```python
from build123d import *

# Parameters (mm, degrees)
ESQUISSE2_R                  = 1.5
ENL_V_MAT_EXTRU_1_DEPTH      = 15.5
ENL_V_MAT_EXTRU_1_DEPTH_BACK = 15.5
ESQUISSE3_R                  = 1.5
ENL_V_MAT_EXTRU_2_DEPTH      = 15.5000001
ENL_V_MAT_EXTRU_2_DEPTH_BACK = 15.5000001
CONG_1_R                     = 2
CONG_2_R                     = 1
CHANFREIN1_SIZE              = 1


with BuildPart() as part:
    # Esquisse1 → Révolution1 (revolve)
    with BuildSketch(Plane(origin=(0, 0, 0), x_dir=(0, 0, -1), z_dir=(1, 0, 0))):
        Polygon((-45, 11), (-45, 7), (-50, 7), (-50, 14.5), (50, 14.5), (50, 11), align=None)
    revolve(axis=Axis((0, 0, 50), (0, 0, -1)))

    # Esquisse2 → Enlèv. mat.-Extru.1 (cut, two sides)
    with BuildSketch(Plane(origin=(0, 0, 0), x_dir=(0, 0, -1), z_dir=(1, 0, 0))) as enl_v_mat_extru_1_sk:
        with Locations((39.5, 0)):
            Circle(ESQUISSE2_R)
    extrude(amount=ENL_V_MAT_EXTRU_1_DEPTH, mode=Mode.SUBTRACT)
    extrude(enl_v_mat_extru_1_sk.sketch, amount=-ENL_V_MAT_EXTRU_1_DEPTH_BACK, mode=Mode.SUBTRACT)

    # Esquisse3 → Enlèv. mat.-Extru.2 (cut, two sides)
    with BuildSketch(Plane(origin=(0, 0, 0), x_dir=(1, 0, 0), z_dir=(0, 1, 0))) as enl_v_mat_extru_2_sk:
        with Locations((0, 45.5)):
            Circle(ESQUISSE3_R)
    extrude(amount=ENL_V_MAT_EXTRU_2_DEPTH, mode=Mode.SUBTRACT)
    extrude(enl_v_mat_extru_2_sk.sketch, amount=-ENL_V_MAT_EXTRU_2_DEPTH_BACK, mode=Mode.SUBTRACT)

    # Congé1
    cong_1_edges = [part.edges().sort_by_distance(p)[0] for p in [
        (0, -11, 45),
    ]]
    fillet(cong_1_edges, radius=CONG_1_R)

    # Congé2
    cong_2_edges = [part.edges().sort_by_distance(p)[0] for p in [
        (0, -7, 45),
    ]]
    fillet(cong_2_edges, radius=CONG_2_R)

    # Chanfrein1
    chanfrein1_edges = [part.edges().sort_by_distance(p)[0] for p in [
        (0, -14.5, 50),
        (0, -14.5, -50),
    ]]
    chamfer(chanfrein1_edges, length=CHANFREIN1_SIZE)


solid = part.part
```
The listing builds one solid part. Answer for the finished solid, in the listing's coordinates (mm). A direction names the side the tool comes from. Round coordinates to 2 decimals unless told otherwise and drop trailing zeros. Write each loop counter-clockwise with the first axis right and the second up, starting at its lowest first coordinate (ties: lowest second). Pieces come first, ordered by that corner, then holes. Notation, with made-up numbers: (40.25, -4) -> (91.25, -4) arc R16 ccw to (91.25, 18) -> close; hole circle Ø9 at (-19.75, -13.5). An arc over 180 degrees is marked (long way). Answer as a JSON object with one key per item and string values. Group by question number.
Q1. Which of the six approach directions +Z, -Z, +X, -X, +Y, -Y give full straight-line access (tool end or side, diameter ignored) to faces 5 (the face through (12.7, -0.9, -38.3)), 6 (the face through (-4.213, 10.161, -2.849))?
Q2. Determine the mould class of faces 1 (the face through (-12.7, -0.9, -38.3)), 2 (the face through (-10, -5, -50)), 3 (the face through (0, 13, -44)), 4 (the face through (-6, -6, 50)) for opening direction Z: pulls with the +Z half, pulls with the -Z half, needs draft (parallel to the pull), parting line crosses it, or undercut.
Q3. Each of these flat-tipped pins is pushed along its axis until it touches: pin 1 Ø1.5 at (y, z) = (-8.5, 3) entering from +X; pin 2 Ø1 at (y, z) = (4.5, 26) entering from -X; pin 3 Ø1.5 at (x, z) = (-5, -0.5) entering from +Y. Where does it stop, or does it pass through?
Q4. Section C-C (z = -39.5) is taken. Write down the section's boundary in (x, y), plus the area to 3 significant figures.
Q5. Section A-A (x = 0) is taken. Write down the section's boundary in (y, z), plus the area to 3 significant figures.
Q6. Straight lines are drawn through the part: line 1 along Z through (x, y) = (-7.25, -5); line 2 along Y through (x, z) = (-0.5, -25.5); line 3 along X through (y, z) = (7, 29). For each, find the intervals that lie inside material, in ascending order.
Q7. Section D-D (z = 0.5) is taken. Write down the section's boundary in (x, y).
Q8. Section B-B (y = 0) is taken. Write down the section's boundary in (x, z).
Check values:
{
 "1": {"face 5": "+X, -X", "face 6": "-Z"},
 "2": {"face 1": "undercut", "face 2": "pulls with the -Z half", "face 3": "undercut", "face 4": "pulls with the +Z half"},
 "3": {"pin 1": "x = 12.26", "pin 2": "x = -13.94", "pin 3": "y = 13.86"},
 "4": {"outline": "(-14.42, -1.5) arc R14.5 ccw to (14.42, -1.5) -> (10.9, -1.5) arc R11 cw to (-10.9, -1.5) -> close; (-14.42, 1.5) -> (-10.9, 1.5) arc R11 cw to (10.9, 1.5) -> (14.42, 1.5) arc R14.5 ccw to start", "area": "259 mm^2"},
 "5": {"outline": "(-14.5, -49) -> (-13.5, -50) -> (-11, -50) -> (-11, -47) -> (-14.5, -47) -> close; (-14.5, -44) -> (-11, -44) -> (-11, 43) arc R2 cw to (-9, 45) -> (-8, 45) arc R1 ccw to (-7, 46) -> (-7, 50) -> (-13.5, 50) -> (-14.5, 49) -> close; (7, 46) arc R1 ccw to (8, 45) -> (9, 45) arc R2 cw to (11, 43) -> (11, -44) -> (14.5, -44) -> (14.5, 49) -> (13.5, 50) -> (7, 50) -> close; (11, -50) -> (13.5, -50) -> (14.5, -49) -> (14.5, -47) -> (11, -47) -> close", "area": "718 mm^2"},
 "6": {"line 1": "45 to 50", "line 2": "-14.49 to -10.99, 10.99 to 14.49", "line 3": "-12.7 to -8.49, 8.49 to 12.7"},
 "7": {"outline": "circle Ø29 at (0, 0); hole circle Ø22 at (0, 0)"},
 "8": {"outline": "(-14.5, -49) -> (-13.5, -50) -> (-11, -50) -> (-11, -41) -> (-14.5, -41) -> close; (-14.5, -38) -> (-11, -38) -> (-11, 43) arc R2 cw to (-9, 45) -> (-8, 45) arc R1 ccw to (-7, 46) -> (-7, 50) -> (-13.5, 50) -> (-14.5, 49) -> close; (7, 46) arc R1 ccw to (8, 45) -> (9, 45) arc R2 cw to (11, 43) -> (11, -38) -> (14.5, -38) -> (14.5, 49) -> (13.5, 50) -> (7, 50) -> close; (11, -50) -> (13.5, -50) -> (14.5, -49) -> (14.5, -41) -> (11, -41) -> close"}
}
